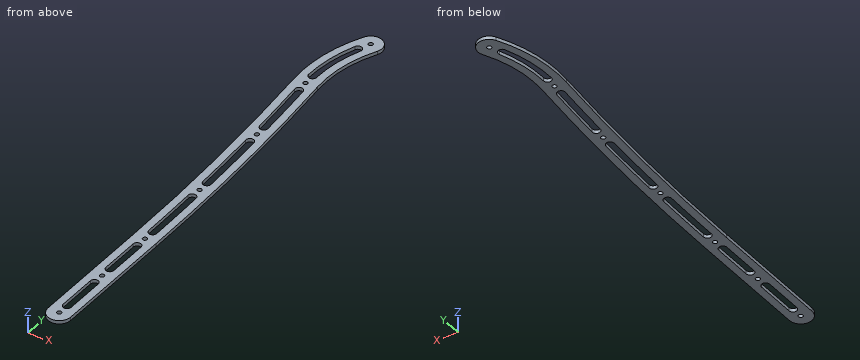
```python
from build123d import *

# Parameters (mm, degrees)
SKETCH_1_R          = 1.95
EXTRUDE_2_DEPTH     = 3
SKETCH_3_R          = 1.95
CUT_EXTRUDE_1_DEPTH = 411.642233029
CUT_EXTRUDE_2_DEPTH = 411.642233029


with BuildPart() as part:
    # 草图1 → 凸台-拉伸2 (new body)
    with BuildSketch(Plane.XY):
        with BuildLine():
            Line((-10, -290), (-10, -400))
            ThreePointArc((-10, -400), (0, -410), (10, -400))
            Line((10, -400), (10, -290))
            ThreePointArc((10, -290), (6.964883906, -177.395762041), (-2.13165062, -65.118518595))
            ThreePointArc((-2.13165062, -65.118518595), (-1.001742213, -34.015540789), (8.921943266, -4.516517282))
            ThreePointArc((8.921943266, -4.516517282), (4.516517282, 8.921943266), (-8.921943266, 4.516517282))
            ThreePointArc((-8.921943266, 4.516517282), (-20.677134638, -30.426817765), (-22.015577858, -67.27013138))
            ThreePointArc((-22.015577858, -67.27013138), (-13.006076822, -178.473132736), (-10, -290))
        make_face()
        Circle(SKETCH_1_R, mode=Mode.SUBTRACT)
        with Locations((0, -400)):
            Circle(SKETCH_1_R, mode=Mode.SUBTRACT)
    extrude(amount=EXTRUDE_2_DEPTH)

    # 草图3 → 切除-拉伸1 (cut, through all)
    with BuildSketch(Plane.XY.offset(3)):
        with Locations((-12.073614239, -66.194324988)):
            Circle(SKETCH_3_R)
        with Locations((0, -290)):
            Circle(SKETCH_3_R)
        with Locations((0, -345)):
            Circle(SKETCH_3_R)
        with Locations((-5.546108146, -138.194324988)):
            Circle(SKETCH_3_R)
        with Locations((-1.246315893, -218)):
            Circle(SKETCH_3_R)
    extrude(amount=-CUT_EXTRUDE_1_DEPTH, mode=Mode.SUBTRACT)

    # 草图4 → 切除-拉伸2 (cut, through all)
    with BuildSketch(Plane.XY.offset(3)):
        with BuildLine():
            Line((3.5, -300), (3.5, -335))
            ThreePointArc((3.5, -335), (0, -338.5), (-3.5, -335))
            Line((-3.5, -335), (-3.5, -300))
            ThreePointArc((-3.5, -300), (0, -296.5), (3.5, -300))
        make_face()
        with BuildLine():
            Line((3.5, -355), (3.5, -390))
            ThreePointArc((3.5, -390), (0, -393.5), (-3.5, -390))
            Line((-3.5, -390), (-3.5, -355))
            ThreePointArc((-3.5, -355), (0, -351.5), (3.5, -355))
        make_face()
        with BuildLine():
            ThreePointArc((-7.748753127, -8.714910959), (-14.36874553, -32.070657967), (-16.228058971, -56.275165217))
            ThreePointArc((-16.228058971, -56.275165217), (-12.648152458, -59.693391271), (-9.229926404, -56.113484758))
            ThreePointArc((-9.229926404, -56.113484758), (-7.477411831, -33.29928315), (-1.237671449, -11.285089041))
            ThreePointArc((-1.237671449, -11.285089041), (-3.208123247, -6.744459161), (-7.748753127, -8.714910959))
        make_face()
        with BuildLine():
            ThreePointArc((-2.812608819, -127.922101985), (-5.01013796, -101.863544894), (-7.534506265, -75.83461682))
            ThreePointArc((-7.534506265, -75.83461682), (-11.375681082, -72.712858338), (-14.497439565, -76.554033155))
            ThreePointArc((-14.497439565, -76.554033155), (-11.981551023, -102.495525828), (-9.79140374, -128.46654799))
            ThreePointArc((-9.79140374, -128.46654799), (-6.029783277, -131.683722448), (-2.812608819, -127.922101985))
        make_face()
        with BuildLine():
            ThreePointArc((1.880579751, -207.862042625), (0.482482294, -177.897281403), (-1.346806184, -147.955750125))
            ThreePointArc((-1.346806184, -147.955750125), (-5.077240441, -144.702465593), (-8.330524974, -148.43289985))
            ThreePointArc((-8.330524974, -148.43289985), (-6.507381374, -178.273852657), (-5.113980353, -208.137957375))
            ThreePointArc((-5.113980353, -208.137957375), (-1.478742925, -211.497280052), (1.880579751, -207.862042625))
        make_face()
        with BuildLine():
            ThreePointArc((3.475925039, -279.98317593), (3.187918187, -253.936615897), (2.574358276, -227.895690765))
            ThreePointArc((2.574358276, -227.895690765), (-1.028396268, -224.501554691), (-4.422532343, -228.104309235))
            ThreePointArc((-4.422532343, -228.104309235), (-3.81103348, -254.057758666), (-3.523994089, -280.01682407))
            ThreePointArc((-3.523994089, -280.01682407), (-0.007210455, -283.499959564), (3.475925039, -279.98317593))
        make_face()
    extrude(amount=-CUT_EXTRUDE_2_DEPTH, mode=Mode.SUBTRACT)


solid = part.part
```
Can you work these out from the model? Positions are in its coordinate system, mm. Round coordinates to 2 decimals unless told otherwise and drop trailing zeros. Loops run counter-clockwise (first coordinate to the right, second up) from the corner with the lowest first, then second, coordinate; pieces in that order, holes last. Notation, with made-up numbers: M 85,-8.75 L 127,-8.75 A36 ccw 127,25.25 Z; hole C -11,75 d1. An arc over 180 degrees is marked long. Answer as a JSON object with one key per item and string values. Group by question number.
Q1. Imagine slicing it at B-B, the plane y = -47. Please give me the cut outline in (x, z).
Q2. Will this pin go through, and if not, where does the flat tip stop? pin 1 (1.5 mm diameter, centred on y = -323.5, z = 1.5, fed in from -X).
Q3. Please list where these lines run through material, in increasing order: L1, parallel to X at y = -290, z = 1.9; L2, parallel to X at y = -307, z = 1.05; L3, parallel to X at y = -286, z = 1.75.
Q4. Imagine slicing it at A-A, the plane y = -305. Please give me the cut outline in (x, z).
Q5. Imagine slicing it at C-C, the plane z = 1.85. Count the separate pieces of the cut face and the enclosed holes in it, then the cut area to 3 significant figures.
Findings:
{
 "1": {"outline": "M -22.6,0 L -16.09,0 L -16.09,3 L -22.6,3 Z; M -9.08,0 L -2.57,0 L -2.57,3 L -9.08,3 Z"},
 "2": {"pin 1": "stops at x = -10"},
 "3": {"L1": "x = -10 to -1.95, 1.95 to 10", "L2": "x = -10 to -3.5, 3.5 to 10", "L3": "x = -10 to 10"},
 "4": {"outline": "M -10,0 L -3.5,0 L -3.5,3 L -10,3 Z; M 3.5,0 L 10,0 L 10,3 L 3.5,3 Z"},
 "5": {"separate pieces": "1", "enclosed holes": "13", "area": "6,080 mm2"}
}
